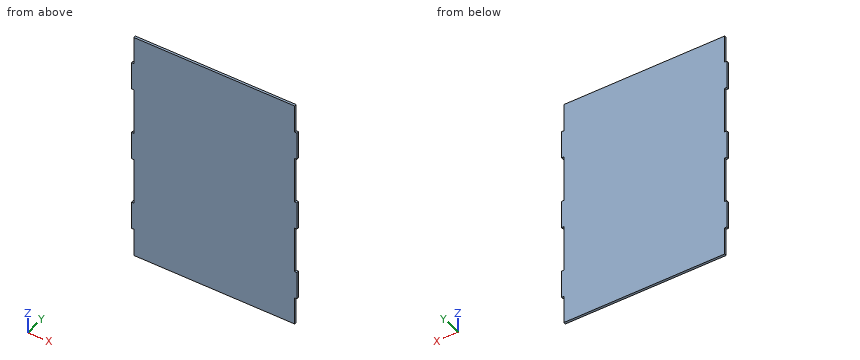
```python
from build123d import *

# Parameters (mm, degrees)
SKETCH1_W           = 226
SKETCH1_H           = 332.7
BOSS_EXTRUDE1_DEPTH = 3.175
SKETCH2_W           = 3.175
SKETCH2_H           = 40
BOSS_EXTRUDE2_DEPTH = 3.175
LPATTERN1_COUNT     = 3
LPATTERN1_PITCH     = 106.35


with BuildPart() as part:
    # Sketch1 → Boss-Extrude1 (new body)
    with BuildSketch(Plane(origin=(0, 0, 0), x_dir=(1, 0, 0), z_dir=(0, 1, 0))):
        with Locations((113, -166.35)):
            Rectangle(SKETCH1_W, SKETCH1_H)
    extrude(amount=BOSS_EXTRUDE1_DEPTH)

    # Sketch2 → Boss-Extrude2 (add)
    with BuildSketch(Plane(origin=(0, 3.175, 0), x_dir=(1, 0, 0), z_dir=(0, 1, 0))):
        with Locations((-1.5875, -60)):
            Rectangle(SKETCH2_W, SKETCH2_H)
        with Locations((227.5875, -60)):
            Rectangle(SKETCH2_W, SKETCH2_H)
    boss_extrude2 = extrude(amount=-BOSS_EXTRUDE2_DEPTH)

    # LPattern1: Boss-Extrude2 ×3
    with Locations(*[(0, 0, i * LPATTERN1_PITCH) for i in range(1, LPATTERN1_COUNT)]):
        add(boss_extrude2)


solid = part.part
```
Work out the finished part from the listing and answer in its coordinate system (mm). Give positions to 0.01 mm unless a question says otherwise; leave off trailing zeros. Write each loop counter-clockwise with the first axis right and the second up, starting at its lowest first coordinate (ties: lowest second). Pieces come first, ordered by that corner, then holes.
(1) The part is cut by section B-B on z = 240. Write down the section's boundary in (x, y) (3 decimals), plus the area to 3 significant figures.
Final values:
outline: (0, 0) - (226, 0) - (226, 3.175) - (0, 3.175) - close
area: 718 mm2
(2) Flat-ended cylindrical pins translate along their axes: pin 1 Ø1 at (x, y) = (228, 1) entering from -Z; pin 2 Ø1.6 at (x, y) = (-2.5, 1.5) entering from +Z; pin 3 Ø1.6 at (y, z) = (2, 22) entering from +X. Find the tip coordinate at first contact, or state that the pin passes through.
Final values:
pin 1: stops at z = 40
pin 2: stops at z = 292.7
pin 3: stops at x = 226
(3) A straight line is drawn through the part: line 1 (X direction, y = 2.7, z = 197.5). Find the intervals that lie inside material, in ascending order.
Final values:
line 1: x = 0 to 226
(4) The part is cut by section A-A on y = 1.3. Write down the section's boundary in (x, z) (3 decimals).
Final values:
outline: (-3.175, 40) - (0, 40) - (0, 0) - (226, 0) - (226, 40) - (229.175, 40) - (229.175, 80) - (226, 80) - (226, 146.35) - (229.175, 146.35) - (229.175, 186.35) - (226, 186.35) - (226, 252.7) - (229.175, 252.7) - (229.175, 292.7) - (226, 292.7) - (226, 332.7) - (0, 332.7) - (0, 292.7) - (-3.175, 292.7) - (-3.175, 252.7) - (0, 252.7) - (0, 186.35) - (-3.175, 186.35) - (-3.175, 146.35) - (0, 146.35) - (0, 80) - (-3.175, 80) - close
